Read the model definition and answer for the solid it produces. Units are mm, in the model's axes. A direction names the side the tool comes from. Coordinates: 2 decimals unless noted, no trailing zeros. Write each loop counter-clockwise with the first axis right and the second up, starting at its lowest first coordinate (ties: lowest second). Pieces come first, ordered by that corner, then holes. Notation, with made-up numbers: (2, 44.5) -> (24, 44.5) arc R34 ccw to (24, 79.5) -> close; hole circle Ø3 at (-26.75, -25). An arc over 180 degrees is marked (long way). Return JSON: item names as keys, results as strings.
from build123d import *

# Parameters (mm, degrees)
SKETCH1_R           = 10.5
BOSS_EXTRUDE1_DEPTH = 5


with BuildPart() as part:
    # Sketch1 → Boss-Extrude1 (new body)
    with BuildSketch(Plane.XY):
        with BuildLine():
            ThreePointArc((-60, 40), (-58.56615935, 31.485082808), (-54.422783478, 23.909322108))
            Line((-54.422783478, 23.909322108), (-16.678178701, -15.837877232))
            ThreePointArc((-16.678178701, -15.837877232), (0, -23), (16.678178701, -15.837877232))
            Line((16.678178701, -15.837877232), (54.422783478, 23.909322108))
            ThreePointArc((54.422783478, 23.909322108), (58.56615935, 31.485082808), (60, 40))
            ThreePointArc((60, 40), (0, 100), (-60, 40))
        make_face()
        with Locations((-32.5, 40)):
            Circle(SKETCH1_R, mode=Mode.SUBTRACT)
        with BuildLine():
            Line((-8.701658453, -8.263240295), (-21.404458824, 5.113525511))
            ThreePointArc((-21.404458824, 5.113525511), (-26.35176104, 17.421416266), (-21.523623248, 29.77653907))
            ThreePointArc((-21.523623248, 29.77653907), (-17.604326655, 41.766045188), (-24.218531469, 52.506689369))
            ThreePointArc((-24.218531469, 52.506689369), (-32.255432897, 68.469423949), (-22.572828784, 83.491003675))
            ThreePointArc((-22.572828784, 83.491003675), (0, 89), (22.572828784, 83.491003675))
            ThreePointArc((22.572828784, 83.491003675), (32.255432897, 68.469423949), (24.218531469, 52.506689369))
            ThreePointArc((24.218531469, 52.506689369), (17.604326655, 41.766045188), (21.523623248, 29.77653907))
            ThreePointArc((21.523623248, 29.77653907), (26.35176104, 17.421416266), (21.404458824, 5.113525511))
            Line((21.404458824, 5.113525511), (8.701658453, -8.263240295))
            ThreePointArc((8.701658453, -8.263240295), (0, -12), (-8.701658453, -8.263240295))
        make_face(mode=Mode.SUBTRACT)
        with Locations((32.5, 40)):
            Circle(SKETCH1_R, mode=Mode.SUBTRACT)
    extrude(amount=BOSS_EXTRUDE1_DEPTH)


solid = part.part
1. The part is cut by section A-A (x = 0). Determine the outline of the cut face in (y, z).
Taken from the geometry:
{"outline": "(-23, 0) -> (-12, 0) -> (-12, 5) -> (-23, 5) -> close; (89, 0) -> (100, 0) -> (100, 5) -> (89, 5) -> close"}
2. Flat-ended cylindrical pins translate along their axes: pin 1 Ø1 at (x, z) = (4.5, 3.5) entering from -Y; pin 2 Ø17 at (x, y) = (32.5, 40) entering from +Z; pin 3 Ø3 at (y, z) = (12, 4) entering from -X; pin 4 Ø1 at (x, z) = (30.5, 3.5) entering from +Y. Find the tip coordinate at first contact, or state that the pin passes through.
Taken from the geometry:
{"pin 1": "stops at y = -22.65", "pin 2": "passes through", "pin 3": "stops at x = -44.54", "pin 4": "stops at y = 91.96"}
3. The part is cut by section B-B (y = 56). Determine the outline of the cut face in (x, z).
Taken from the geometry:
{"outline": "(-57.83, 0) -> (-28.12, 0) -> (-28.12, 5) -> (-57.83, 5) -> close; (28.12, 0) -> (57.83, 0) -> (57.83, 5) -> (28.12, 5) -> close"}
4. A tool of negligible diameter and unlimited length cuts with its end or side. For faces 4 (the face through (-58.606, 31.6, 2.465)), 5 (the face through (-14.96, -1.67, 2.46)), from which of +Z, -Z, +X, -X, +Y, -Y can it reach the whole face along a straight path? Write none if from no direction.
Taken from the geometry:
{"face 4": "+Z, -Z, -X, -Y", "face 5": "+Z, -Z"}
5. The part is cut by section C-C (z = 3.65). Determine the outline of the cut face in (x, y), then the cut area to 3 significant figures.
Taken from the geometry:
{"outline": "(-60, 40) arc R26 ccw to (-54.42, 23.91) -> (-16.68, -15.84) arc R23 ccw to (16.68, -15.84) -> (54.42, 23.91) arc R26 ccw to (60, 40) arc R60 ccw to start; hole circle Ø21 at (-32.5, 40); hole (-24.22, 52.51) arc R15 cw to (-21.52, 29.78) arc R18 ccw to (-21.4, 5.11) -> (-8.7, -8.26) arc R12 ccw to (8.7, -8.26) -> (21.4, 5.11) arc R18 ccw to (21.52, 29.78) arc R15 cw to (24.22, 52.51) arc R18 ccw to (22.57, 83.49) arc R49 ccw to (-22.57, 83.49) arc R18 ccw to start; hole circle Ø21 at (32.5, 40)", "area": "5,280 mm2"}
6. Consider L1, parallel to X at y = 44.5, z = 1.6; L2, parallel to X at y = 49, z = 4.05; L3, parallel to Y at x = 6.5, z = 2.45. Determine where each line is inside the solid, lowest interval first.
Taken from the geometry:
{"L1": "x = -59.83 to -41.99, -23.01 to -18.19, 18.19 to 23.01, 41.99 to 59.83", "L2": "x = -59.32 to -37.91, -27.09 to -20.5, 20.5 to 27.09, 37.91 to 59.32", "L3": "y = -22.06 to -10.09, 88.57 to 99.65"}
7. For a pull along Y with two mould halves and no side action, classify faces 1 (the face through (26, 53, 0)), 2 (the face through (17.627, 41.947, 2.465)), 3 (the face through (0, -23, 2)) as +Y half, -Y half, draft (parallel to the pull), parting line (faces both ways), or undercut.
Taken from the geometry:
{"face 1": "draft", "face 2": "undercut", "face 3": "-Y half"}
8. The part is cut by section D-D (x = -50). Determine the outline of the cut face in (y, z).
Taken from the geometry:
{"outline": "(19.25, 0) -> (73.17, 0) -> (73.17, 5) -> (19.25, 5) -> close"}
